from build123d import *

# Parameters (mm, degrees)
SKETCH1_W           = 450
SKETCH1_H           = 450
BOSS_EXTRUDE1_DEPTH = 5
BOSS_EXTRUDE2_DEPTH = 7.48
BOSS_EXTRUDE3_DEPTH = 7.48
SKETCH6_W           = 450
SKETCH6_H           = 450
CUT_EXTRUDE1_DEPTH  = 5
SKETCH7_R           = 11
SKETCH7_R_2         = 2.5
CUT_EXTRUDE2_DEPTH  = 10
SKETCH8_R           = 2.5
CUT_EXTRUDE4_DEPTH  = 10


# Read off the part's stored shape, not the designer's step: Boss-Extrude2
with BuildPart() as part:
    # Sketch1 → Boss-Extrude1 (new body)
    with BuildSketch(Plane(origin=(0, 0, 0), x_dir=(0, 0, -1), z_dir=(1, 0, 0))):
        Rectangle(SKETCH1_W, SKETCH1_H)
    extrude(amount=BOSS_EXTRUDE1_DEPTH)

    # Boss-Extrude2 outline → Boss-Extrude2 (add)
    with BuildSketch(Plane(origin=(5, 0, 0), x_dir=(0, 0, -1), z_dir=(1, 0, 0))):
        with BuildLine():
            Line((-164.971757583, 8.09), (-209.152698388, 8.09))
            ThreePointArc((-209.152698388, 8.09), (-209.3091, 0), (-209.152698388, -8.09))
            Line((-209.152698388, -8.09), (-164.971757583, -8.09))
            ThreePointArc((-164.971757583, -8.09), (-116.792827049, -116.792827049), (-8.09, -164.971757583))
            Line((-8.09, -164.971757583), (-8.09, -209.152698388))
            ThreePointArc((-8.09, -209.152698388), (0, -209.3091), (8.09, -209.152698388))
            Line((8.09, -209.152698388), (8.09, -164.971757583))
            ThreePointArc((8.09, -164.971757583), (116.792827049, -116.792827049), (164.971757583, -8.09))
            Line((164.971757583, -8.09), (209.152698388, -8.09))
            ThreePointArc((209.152698388, -8.09), (209.3091, 0), (209.152698388, 8.09))
            Line((209.152698388, 8.09), (164.971757583, 8.09))
            ThreePointArc((164.971757583, 8.09), (116.792827049, 116.792827049), (8.09, 164.971757583))
            Line((8.09, 164.971757583), (8.09, 209.152698388))
            ThreePointArc((8.09, 209.152698388), (0, 209.3091), (-8.09, 209.152698388))
            Line((-8.09, 209.152698388), (-8.09, 164.971757583))
            ThreePointArc((-8.09, 164.971757583), (-116.792827049, 116.792827049), (-164.971757583, 8.09))
        make_face()
        with BuildLine():
            Line((148.770198629, 8.09), (104.538333308, 8.09))
            ThreePointArc((104.538333308, 8.09), (104.8509, 0), (104.538333308, -8.09))
            Line((104.538333308, -8.09), (148.770198629, -8.09))
            ThreePointArc((148.770198629, -8.09), (105.351839329, -105.351839329), (8.09, -148.770198629))
            Line((8.09, -148.770198629), (8.09, -104.538333308))
            ThreePointArc((8.09, -104.538333308), (0, -104.8509), (-8.09, -104.538333308))
            Line((-8.09, -104.538333308), (-8.09, -148.770198629))
            ThreePointArc((-8.09, -148.770198629), (-105.351839329, -105.351839329), (-148.770198629, -8.09))
            Line((-148.770198629, -8.09), (-104.538333308, -8.09))
            ThreePointArc((-104.538333308, -8.09), (-104.8509, 0), (-104.538333308, 8.09))
            Line((-104.538333308, 8.09), (-148.770198629, 8.09))
            ThreePointArc((-148.770198629, 8.09), (-105.351839329, 105.351839329), (-8.09, 148.770198629))
            Line((-8.09, 148.770198629), (-8.09, 104.538333308))
            ThreePointArc((-8.09, 104.538333308), (0, 104.8509), (8.09, 104.538333308))
            Line((8.09, 104.538333308), (8.09, 148.770198629))
            ThreePointArc((8.09, 148.770198629), (105.351839329, 105.351839329), (148.770198629, 8.09))
        make_face(mode=Mode.SUBTRACT)
    extrude(amount=BOSS_EXTRUDE2_DEPTH)

    # Sketch5 → Boss-Extrude3 (add)
    with BuildSketch(Plane(origin=(5, 0, 0), x_dir=(0, 0, -1), z_dir=(1, 0, 0))):
        with BuildLine():
            Line((-19.319547743, 8.09), (-104.275748565, 8.09))
            ThreePointArc((-104.275748565, 8.09), (-104.5891, 0), (-104.275748565, -8.09))
            Line((-104.275748565, -8.09), (-19.319547743, -8.09))
            ThreePointArc((-19.319547743, -8.09), (0, -20.945), (19.319547743, -8.09))
            Line((19.319547743, -8.09), (104.275748565, -8.09))
            ThreePointArc((104.275748565, -8.09), (104.5891, 0), (104.275748565, 8.09))
            Line((104.275748565, 8.09), (19.319547743, 8.09))
            ThreePointArc((19.319547743, 8.09), (0, 20.945), (-19.319547743, 8.09))
        make_face()
    extrude(amount=BOSS_EXTRUDE3_DEPTH)

    # Sketch6 → Cut-Extrude1 (cut)
    with BuildSketch(Plane.ZY):
        Rectangle(SKETCH6_W, SKETCH6_H)
    extrude(amount=-CUT_EXTRUDE1_DEPTH, mode=Mode.SUBTRACT)


with BuildPart() as cut_extrude1_piece_1:
    # of the separate pieces the step leaves, piece 1, a body of its own (cut_extrude1_pieces)
    add(part.part.solids().sort_by_distance((5, 209.152698388, 8.09))[0])


with BuildPart() as cut_extrude1_piece_2:
    # of the separate pieces the step leaves, piece 2, a body of its own (cut_extrude1_pieces)
    add(part.part.solids().sort_by_distance((5, 8.09, -104.275748565))[0])


with BuildPart() as cut_extrude2_tool:
    # Sketch7 → Cut-Extrude2 (new body)
    with BuildSketch(Plane(origin=(12.48, 0, 0), x_dir=(0, 0, -1), z_dir=(1, 0, 0))):
        Circle(SKETCH7_R)
        with Locations((-183.1891, 0)):
            Circle(SKETCH7_R_2)
        with Locations((-130.9659, 0)):
            Circle(SKETCH7_R_2)
        with Locations((0, -183.1891)):
            Circle(SKETCH7_R_2)
        with Locations((0, -130.9659)):
            Circle(SKETCH7_R_2)
        with Locations((183.1891, 0)):
            Circle(SKETCH7_R_2)
        with Locations((52.3, 0)):
            Circle(SKETCH7_R_2)
        with Locations((-52.295, 0)):
            Circle(SKETCH7_R_2)
        with Locations((0, 183.1891)):
            Circle(SKETCH7_R_2)
        with Locations((0, 130.9659)):
            Circle(SKETCH7_R_2)
        with BuildLine():
            Line((-3, 13.8), (-3, 10.583005244))
            ThreePointArc((-3, 10.583005244), (0, 11), (3, 10.583005244))
            Line((3, 10.583005244), (3, 13.8))
            Line((3, 13.8), (-3, 13.8))
        make_face()
        with Locations((130.9659, 0)):
            Circle(SKETCH7_R_2)
    extrude(amount=-CUT_EXTRUDE2_DEPTH)


with BuildPart() as cut_extrude1_piece_1_1:
    add(cut_extrude1_piece_1.part)

    # Cut-Extrude2: cut by cut_extrude2_tool
    add(cut_extrude2_tool.part, mode=Mode.SUBTRACT)


with BuildPart() as cut_extrude1_piece_2_1:
    add(cut_extrude1_piece_2.part)

    # Cut-Extrude2: cut by cut_extrude2_tool
    add(cut_extrude2_tool.part, mode=Mode.SUBTRACT)

    # Sketch8 → Cut-Extrude4 (cut)
    with BuildSketch(Plane(origin=(12.48, 0, 0), x_dir=(0, 0, -1), z_dir=(1, 0, 0))):
        with BuildLine():
            ThreePointArc((19.319547743, 8.09), (0, 20.945), (-19.319547743, 8.09))
            Line((-19.319547743, 8.09), (-104.275748565, 8.09))
            ThreePointArc((-104.275748565, 8.09), (-104.5891, 0), (-104.275748565, -8.09))
            Line((-104.275748565, -8.09), (-19.319547743, -8.09))
            ThreePointArc((-19.319547743, -8.09), (0, -20.945), (19.319547743, -8.09))
            Line((19.319547743, -8.09), (104.275748565, -8.09))
            ThreePointArc((104.275748565, -8.09), (104.5891, 0), (104.275748565, 8.09))
            Line((104.275748565, 8.09), (19.319547743, 8.09))
        make_face()
        with Locations((-52.295, 0)):
            Circle(SKETCH8_R, mode=Mode.SUBTRACT)
        with Locations((52.3, 0)):
            Circle(SKETCH8_R, mode=Mode.SUBTRACT)
        with BuildLine():
            Line((3, 13.8), (3, 10.583005244))
            ThreePointArc((3, 10.583005244), (0, -11), (-3, 10.583005244))
            Line((-3, 10.583005244), (-3, 13.8))
            Line((-3, 13.8), (3, 13.8))
        make_face(mode=Mode.SUBTRACT)
    extrude(amount=-CUT_EXTRUDE4_DEPTH, mode=Mode.SUBTRACT)


solid = cut_extrude1_piece_1_1.part
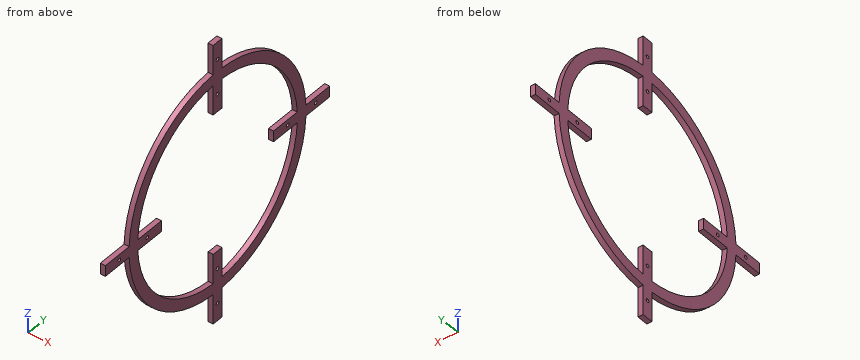
Verification items for the finished model (mm, model axes). Give positions to 0.01 mm unless a question says otherwise; leave off trailing zeros. Order: outer loops, then holes, each group sorted by start corner. A loop starts at its lowest first (then second) coordinate and runs counter-clockwise, first axis right, second up. Notation, with made-up numbers: M 15.5,-34.5 L 47.5,-34.5 A8 ccw 47.5,-26.5 Z; hole C 84.25,83 d11. An arc over 180 degrees is marked long. Answer as a JSON object with one key per item and string values. Group by question number.
1) Depth check by flat-ended pin: pin 1 Ø6.5 at (y, z) = (130.97, 0) entering from +X; pin 2 Ø1.5 at (x, y) = (6, 150) entering from -Z; pin 3 Ø3 at (x, z) = (8, 55.5) entering from -Y; pin 4 Ø3.5 at (x, y) = (7, 186.5) entering from +Z. Enter the tip coordinate at first touch or a pass-through.
2) Cross-section at B-B (y = 70.5). Enter the section's corners in (x, z), then the cut area to 3 significant figures.
3) Cross-section at C-C (z = -115). Enter the section's corners in (x, y).
4) Scan lines: line 1 along Y through (x, z) = (7.25, 0); line 2 along Y through (x, z) = (9.5, -114); line 3 along Y through (x, z) = (9, -9). Record each from-to range of solid material in increasing order. Write a range as [from, to].
5) Cross-section at D-D (x = 6.75). Give the number of separate pieces and of enclosed holes in the cut face, then the cut area to 3 significant figures.
6) Cross-section at A-A (z = 73). Enter the section's corners in (x, y), then the cut area to 3 significant figures.
Result sheet:
{
 "1": {"pin 1": "stops at x = 12.48", "pin 2": "stops at z = -70.75", "pin 3": "stops at y = -156.09", "pin 4": "stops at z = 8.09"},
 "2": {"outline": "M 5,-149.37 L 12.48,-149.37 L 12.48,-131.25 L 5,-131.25 Z; M 5,131.25 L 12.48,131.25 L 12.48,149.37 L 5,149.37 Z", "area": "271 mm2"},
 "3": {"outline": "M 5,-118.56 L 12.48,-118.56 L 12.48,-94.73 L 5,-94.73 Z; M 5,-8.09 L 12.48,-8.09 L 12.48,8.09 L 5,8.09 Z; M 5,94.73 L 12.48,94.73 L 12.48,118.56 L 5,118.56 Z"},
 "4": {"line 1": "y = [-209.31, -185.69], [-180.69, -133.47], [-128.47, -104.85], [104.85, 128.47], [133.47, 180.69], [185.69, 209.31]", "line 2": "y = [-119.52, -95.93], [-8.09, 8.09], [95.93, 119.52]", "line 3": "y = [-164.92, -148.72], [148.72, 164.92]"},
 "5": {"separate pieces": "1", "enclosed holes": "9", "area": "21,500 mm2"},
 "6": {"outline": "M 5,-148.16 L 12.48,-148.16 L 12.48,-129.88 L 5,-129.88 Z; M 5,129.88 L 12.48,129.88 L 12.48,148.16 L 5,148.16 Z", "area": "273 mm2"}
}
